from build123d import *

# Parameters (mm, degrees)
SKETCH_1_W                     = 53
SKETCH_1_H                     = 20
EXTRUDE_1_DEPTH                = 50
HOLE_WIZARD_M5_1_D             = 5.25
HOLE_WIZARD_M5_1_DEPTH         = 15
HOLE_WIZARD_M5_1_TIP           = 1.577259125
SKETCH_4_W                     = 5
SKETCH_4_H                     = 20
EXTRUDE_2_DEPTH                = 20
HOLE_WIZARD_M4_1_D             = 4.5
HOLE_WIZARD_M4_1_DEPTH         = 15
HOLE_WIZARD_M4_1_CBORE_D       = 8
HOLE_WIZARD_M4_1_CBORE_DEPTH   = 3
HOLE_WIZARD_M4_1_TIP           = 1.351936393
SKETCH_7_W                     = 5
SKETCH_7_H                     = 20
EXTRUDE_3_DEPTH                = 20
HOLE_WIZARD_M5_1_2_D           = 5.5
HOLE_WIZARD_M5_1_2_DEPTH       = 15
HOLE_WIZARD_M5_1_2_CBORE_D     = 9.5
HOLE_WIZARD_M5_1_2_CBORE_DEPTH = 3
HOLE_WIZARD_M5_1_2_TIP         = 1.652366702
FILLET_1_R                     = 10
SKETCH_10_W                    = 6
SKETCH_10_H                    = 8
SKETCH_10_W_2                  = 7
SKETCH_10_H_2                  = 9.5
CUT_EXTRUDE_1_DEPTH            = 20


with BuildPart() as part:
    # 스케치1 → 보스-돌출1 (new body)
    with BuildSketch(Plane.XY):
        Rectangle(SKETCH_1_W, SKETCH_1_H)
    extrude(amount=EXTRUDE_1_DEPTH)

    # Hole Wizard M5 _ _1
    with Locations(Plane.XY.offset(50)):
        with Locations((20.5, 0), (-20.5, 0)):
            Hole(HOLE_WIZARD_M5_1_D / 2, depth=HOLE_WIZARD_M5_1_DEPTH)
            with Locations((0, 0, -(HOLE_WIZARD_M5_1_DEPTH + HOLE_WIZARD_M5_1_TIP / 2))):  # 118° drill point
                Cone(0, HOLE_WIZARD_M5_1_D / 2, HOLE_WIZARD_M5_1_TIP, mode=Mode.SUBTRACT)

    # 스케치4 → 보스-돌출2 (add)
    with BuildSketch(Plane.ZY.offset(26.5)):
        with Locations((2.5, 0)):
            Rectangle(SKETCH_4_W, SKETCH_4_H)
    extrude(amount=EXTRUDE_2_DEPTH)

    # M4 소켓 머리 캡 나사용 카운터보어1
    with Locations(Plane.XY.offset(5)):
        with Locations((-36.5, 0)):
            CounterBoreHole(HOLE_WIZARD_M4_1_D / 2, HOLE_WIZARD_M4_1_CBORE_D / 2, HOLE_WIZARD_M4_1_CBORE_DEPTH, depth=HOLE_WIZARD_M4_1_DEPTH)
            with Locations((0, 0, -(HOLE_WIZARD_M4_1_DEPTH + HOLE_WIZARD_M4_1_TIP / 2))):  # 118° drill point
                Cone(0, HOLE_WIZARD_M4_1_D / 2, HOLE_WIZARD_M4_1_TIP, mode=Mode.SUBTRACT)

    # 스케치7 → 보스-돌출3 (add)
    with BuildSketch(Plane(origin=(26.5, 0, 0), x_dir=(0, 0, -1), z_dir=(1, 0, 0))):
        with Locations((-2.5, 0)):
            Rectangle(SKETCH_7_W, SKETCH_7_H)
    extrude(amount=EXTRUDE_3_DEPTH)

    # Hole Wizard M5 _ _ _ _ _1 2
    with Locations(Plane.XY.offset(5)):
        with Locations((36.5, 0)):
            CounterBoreHole(HOLE_WIZARD_M5_1_2_D / 2, HOLE_WIZARD_M5_1_2_CBORE_D / 2, HOLE_WIZARD_M5_1_2_CBORE_DEPTH, depth=HOLE_WIZARD_M5_1_2_DEPTH)
            with Locations((0, 0, -(HOLE_WIZARD_M5_1_2_DEPTH + HOLE_WIZARD_M5_1_2_TIP / 2))):  # 118° drill point
                Cone(0, HOLE_WIZARD_M5_1_2_D / 2, HOLE_WIZARD_M5_1_2_TIP, mode=Mode.SUBTRACT)

    # 필렛1
    # the kernel refuses this fillet: 10 mm, written as the material it adds along each edge
    with BuildSketch(Plane(origin=(-26.5, 10, 5), x_dir=(0, 0, 1), z_dir=(0, -1, 0))) as fillet_1_piece_1_section:
        with BuildLine():
            CenterArc((FILLET_1_R, FILLET_1_R), FILLET_1_R, 180, 90)
            Line((0, FILLET_1_R), (0, 0))
            Line((0, 0), (FILLET_1_R, 0))
        make_face()
    fillet_1_piece_1 = extrude(amount=20, mode=Mode.PRIVATE)
    fillet_1_piece_1 = fillet_1_piece_1 - Plane(origin=(-36.5, 0, 7.308851988), x_dir=(1, 0, 0), z_dir=(0, 0, 1)) * Cylinder(4, 81, mode=Mode.PRIVATE)
    add(fillet_1_piece_1)
    with BuildSketch(Plane(origin=(26.5, 10, 5), x_dir=(0, 0, 1), z_dir=(0, -1, 0))) as fillet_1_piece_2_section:
        with BuildLine():
            CenterArc((FILLET_1_R, -FILLET_1_R), FILLET_1_R, 90, 90)
            Line((0, -FILLET_1_R), (0, 0))
            Line((0, 0), (FILLET_1_R, 0))
        make_face()
    fillet_1_piece_2 = extrude(amount=20, mode=Mode.PRIVATE)
    fillet_1_piece_2 = fillet_1_piece_2 - Plane(origin=(36.5, 0, 7.33913119), x_dir=(1, 0, 0), z_dir=(0, 0, 1)) * Cylinder(4.75, 80, mode=Mode.PRIVATE)
    add(fillet_1_piece_2)

    # 스케치10 → 컷-돌출1 (cut)
    with BuildSketch(Plane.XY.offset(5)):
        with Locations((-33.5, 0)):
            Rectangle(SKETCH_10_W, SKETCH_10_H)
        with Locations((33, 0)):
            Rectangle(SKETCH_10_W_2, SKETCH_10_H_2)
    extrude(amount=CUT_EXTRUDE_1_DEPTH, mode=Mode.SUBTRACT)


solid = part.part
Verification items for the finished model (mm, model axes). A direction names the side the tool comes from. Coordinates: 2 decimals unless noted, no trailing zeros. Write each loop counter-clockwise with the first axis right and the second up, starting at its lowest first coordinate (ties: lowest second). Pieces come first, ordered by that corner, then holes. Notation, with made-up numbers: M 1,-8.75 L 25,-8.75 A4 cw 25,-4.75 Z; hole C 14,-20.5 d8. An arc over 180 degrees is marked long. Use CSV: the item, a comma, the result in double quotes.
Q1. Set-up check for faces 1 (the flat face through (-32, -4, 5.6)), 2 (the flat face through (-41, 0, 5)), 3 (the flat face through (29.5, 0, 6)): record each of +Z, -Z, +X, -X, +Y, -Y from which the full face is reachable in a straight line by a thin tool's end or side.
Computed values:
face 1,"+Z, -X"
face 2,"+Z, -X, +Y, -Y"
face 3,"+Z, +X"
Q2. Section check C-C, the plane x = -35.5. Enter the section's corners in (y, z), and give its area (3 significant figures).
Computed values:
outline,"M -10,0 L -2.02,0 L -2.02,2 L -3.87,2 L -3.87,5 L -4,5 L -4,5.05 L -10,5.05 Z; M 2.02,0 L 10,0 L 10,5.05 L 4,5.05 L 4,5 L 3.87,5 L 3.87,2 L 2.02,2 Z"
area,"69.3 mm²"
Q3. Section check A-A, the plane y = -7.75. Enter the section's corners in (x, z), and give its area (3 significant figures).
Computed values:
outline,"M -46.5,0 L 46.5,0 L 46.5,5 L 36.5,5 A10 cw 26.5,15 L 26.5,50 L -26.5,50 L -26.5,15 A10 cw -36.5,5 L -46.5,5 Z"
area,"2,890 mm²"
Q4. Go/stop test with flat-tipped pins: P1, Ø7, axis at x = -36.5, y = 0, coming from the +Z side; P2, Ø4, axis at y = -8, z = 29.5, coming from the +X side; P3, Ø9, axis at x = -36, y = -0.5, coming from the +Z side. Record where each tip stops, or that it passes through.
Computed values:
P1,"z = 2"
P2,"x = 26.5"
P3,"z = 5.57"
Q5. Section check B-B, the plane z = 41. Enter the section's corners in (x, y) (3 decimals).
Computed values:
outline,"M -26.5,-10 L 26.5,-10 L 26.5,10 L -26.5,10 Z; hole C -20.5,0 d5.25; hole C 20.5,0 d5.25"
Q6. Thickness scan on line 1 along X through (y, z) = (0, 3.3); line 2 along X through (y, z) = (0, 46.75) (3 decimals); line 3 along Y through (x, z) = (36.5, 0.55). Record the ranges inside material, lowest first. Write a range as [from, to].
Computed values:
line 1,"[-46.5, -40.5], [-32.5, 31.75], [41.25, 46.5]"
line 2,"[-26.5, -23.125], [-17.875, 17.875], [23.125, 26.5]"
line 3,"[-10, -2.75], [2.75, 10]"
Q7. Section check D-D, the plane z = 30. Enter the section's corners in (x, y).
Computed values:
outline,"M -26.5,-10 L 26.5,-10 L 26.5,10 L -26.5,10 Z"
